Check sheet for the drawn part. Datum: minimum x, y, z corner. Units: mm. Give positions to 0.01 mm unless a question says otherwise; leave off trailing zeros. Order: outer loops, then holes, each group sorted by start corner. A loop starts at its lowest first (then second) coordinate and runs counter-clockwise, first axis right, second up. Notation, with made-up numbers: M 10,37.5 L 30,37.5 A19 ccw 30,63.5 Z; hole C 8,24 d1. An arc over 180 degrees is marked long. One line per question, with ' | ' between items. Start each with the question number.
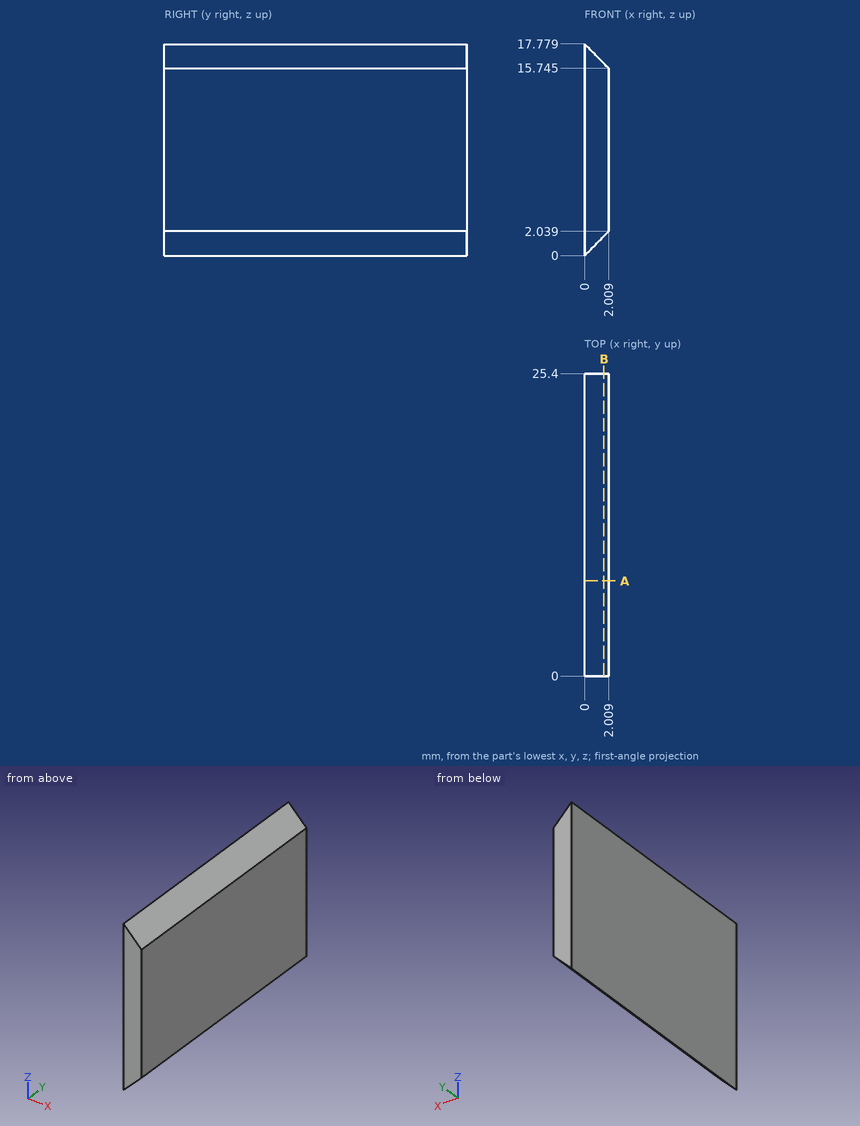
Item 1: Go/stop test with a flat-tipped pin: P1, Ø1, axis at y = 14, z = 15.5, coming from the -X side. Record where the tip stops, or that it passes through.
Item 2: Section check B-B, the plane x = 1.6. Record the cut outline in (y, z).
Item 3: Scan lines: probe 1 along Z at (x, y) = (0.85, 1.5) (1 decimal); probe 2 along Z at (x, y) = (0.35, 15) (1 decimal); probe 3 along X at (y, z) = (7.5, 2). Record each from-to range of solid material in increasing order. Write a range as [from, to].
Item 4: Section check A-A, the plane y = 8. Record the cut outline in (x, z) (1 decimal).
Reported:
1) P1: stops at x = 0
2) outline: M 0,1.62 L 25.4,1.62 L 25.4,16.16 L 0,16.16 Z
3) probe 1: z = [0.9, 16.9] | probe 2: z = [0.4, 17.4] | probe 3: x = [0, 1.97]
4) outline: M 0,0 L 2,2 L 2,15.7 L 0,17.8 Z
